from build123d import *

# Parameters (mm, degrees)
BOSS_EXTRUDE1_DEPTH  = 3.175
SKETCH2_W            = 107.95
SKETCH2_H            = 3.175
CUT_EXTRUDE1_DEPTH   = 355.989990176
SKETCH3_W            = 133.35
SKETCH3_H            = 19.05
CUT_EXTRUDE2_DEPTH   = 355.989990176
FILLET1_R            = 1.5875
CUT_EXTRUDE3_DEPTH   = 355.989990176
LPATTERN1_COUNT      = 2
LPATTERN1_PITCH      = 101.6
LPATTERN1_COUNT_DIR2 = 2
LPATTERN1_PITCH_DIR2 = 146.05
CUT_EXTRUDE4_DEPTH   = 355.989990176
FILLET2_R            = 1.5875


with BuildPart() as part:
    # Sketch1 → Boss-Extrude1 (new body)
    with BuildSketch(Plane(origin=(0, 0, 0), x_dir=(1, 0, 0), z_dir=(0, 1, 0))):
        Polygon((130.175, 0), (158.75, 0), (158.75, 317.5), (0, 317.5), (0, 0), (28.575, 0), (28.575, -3.175), (130.175, -3.175), align=None)
    extrude(amount=BOSS_EXTRUDE1_DEPTH)

    # Sketch2 → Cut-Extrude1 (cut, through all)
    with BuildSketch(Plane(origin=(0, 3.175, 0), x_dir=(1, 0, 0), z_dir=(0, 1, 0))):
        with Locations((79.375, 315.9125)):
            Rectangle(SKETCH2_W, SKETCH2_H)
    extrude(amount=-CUT_EXTRUDE1_DEPTH, mode=Mode.SUBTRACT)

    # Sketch3 → Cut-Extrude2 (cut, through all)
    with BuildSketch(Plane(origin=(0, 3.175, 0), x_dir=(1, 0, 0), z_dir=(0, 1, 0))):
        with Locations((79.375, 57.15)):
            Rectangle(SKETCH3_W, SKETCH3_H)
    extrude(amount=-CUT_EXTRUDE2_DEPTH, mode=Mode.SUBTRACT)

    # Fillet1
    fillet1_edges = [part.edges().sort_by_distance(p)[0] for p in [
        (25.4, 1.5875, -314.325),
        (25.4, 1.5875, -317.5),
        (0, 1.5875, -317.5),
        (0, 1.5875, 0),
        (28.575, 1.5875, 0),
        (28.575, 1.5875, 3.175),
        (130.175, 1.5875, 3.175),
        (130.175, 1.5875, 0),
        (158.75, 1.5875, 0),
        (158.75, 1.5875, -317.5),
        (133.35, 1.5875, -317.5),
        (133.35, 1.5875, -314.325),
    ]]
    fillet(fillet1_edges, radius=FILLET1_R - 0.0001)  # a hair under: the kernel refuses the full size

    # Sketch4 → Cut-Extrude3 (cut, through all)
    with BuildSketch(Plane(origin=(0, 3.175, 0), x_dir=(1, 0, 0), z_dir=(0, 1, 0))):
        with BuildLine():
            Line((4.445, 238.114159312), (4.445, 241.3))
            ThreePointArc((4.445, 241.3), (6.35, 243.205), (8.255, 241.3))
            Line((8.255, 241.3), (8.255, 238.114159312))
            ThreePointArc((8.255, 238.114159312), (6.35, 230.66375), (4.445, 238.114159312))
        make_face()
    cut_extrude3 = extrude(amount=-CUT_EXTRUDE3_DEPTH, mode=Mode.SUBTRACT)

    # LPattern1: Cut-Extrude3 2 × 2
    with Locations(*[(j * LPATTERN1_PITCH_DIR2, 0, i * LPATTERN1_PITCH) for i in range(LPATTERN1_COUNT) for j in range(LPATTERN1_COUNT_DIR2) if (i, j) != (0, 0)]):
        add(cut_extrude3, mode=Mode.SUBTRACT)

    # Sketch5 → Cut-Extrude4 (cut, through all)
    with BuildSketch(Plane(origin=(0, 3.175, 0), x_dir=(1, 0, 0), z_dir=(0, 1, 0))):
        Polygon((139.7, 111.125), (114.3, 85.725), (133.35, 85.725), (139.7, 92.075), align=None)
        Polygon((139.7, 149.225), (76.2, 85.725), (95.25, 85.725), (139.7, 130.175), align=None)
        Polygon((139.7, 187.325), (38.1, 85.725), (57.15, 85.725), (139.7, 168.275), align=None)
        Polygon((19.05, 104.775), (19.05, 85.725), (139.7, 206.375), (139.7, 225.425), align=None)
        Polygon((19.05, 142.875), (19.05, 123.825), (139.7, 244.475), (139.7, 263.525), align=None)
        Polygon((19.05, 180.975), (19.05, 161.925), (139.7, 282.575), (139.7, 295.275), (133.35, 295.275), align=None)
        Polygon((19.05, 219.075), (19.05, 200.025), (114.3, 295.275), (95.25, 295.275), align=None)
        Polygon((19.05, 257.175), (19.05, 238.125), (76.2, 295.275), (57.15, 295.275), align=None)
        Polygon((19.05, 295.275), (19.05, 276.225), (38.1, 295.275), align=None)
    extrude(amount=-CUT_EXTRUDE4_DEPTH, mode=Mode.SUBTRACT)

    # Fillet2
    fillet2_edges = [part.edges().sort_by_distance(p)[0] for p in [
        (19.05, 1.5875, -104.775),
        (139.7, 1.5875, -225.425),
        (139.7, 1.5875, -206.375),
        (19.05, 1.5875, -85.725),
        (19.05, 1.5875, -142.875),
        (139.7, 1.5875, -263.525),
        (139.7, 1.5875, -244.475),
        (19.05, 1.5875, -123.825),
        (95.25, 1.5875, -85.725),
        (76.2, 1.5875, -85.725),
        (139.7, 1.5875, -149.225),
        (139.7, 1.5875, -130.175),
        (57.15, 1.5875, -85.725),
        (38.1, 1.5875, -85.725),
        (139.7, 1.5875, -187.325),
        (139.7, 1.5875, -168.275),
        (19.05, 1.5875, -257.175),
        (57.15, 1.5875, -295.275),
        (76.2, 1.5875, -295.275),
        (19.05, 1.5875, -238.125),
        (19.05, 1.5875, -276.225),
        (19.05, 1.5875, -295.275),
        (38.1, 1.5875, -295.275),
        (19.05, 1.5875, -180.975),
        (133.35, 1.5875, -295.275),
        (139.7, 1.5875, -295.275),
        (139.7, 1.5875, -282.575),
        (19.05, 1.5875, -161.925),
        (19.05, 1.5875, -219.075),
        (95.25, 1.5875, -295.275),
        (114.3, 1.5875, -295.275),
        (19.05, 1.5875, -200.025),
        (133.35, 1.5875, -85.725),
        (114.3, 1.5875, -85.725),
        (139.7, 1.5875, -111.125),
        (139.7, 1.5875, -92.075),
    ]]
    fillet(fillet2_edges, radius=FILLET2_R)


solid = part.part
Can you work these out from the model? Positions are in its coordinate system, mm. Give positions to 0.01 mm unless a question says otherwise; leave off trailing zeros. Loops run counter-clockwise (first coordinate to the right, second up) from the corner with the lowest first, then second, coordinate; pieces in that order, holes last. Notation, with made-up numbers: (69, -3.5) -> (93, -3.5) arc R17 ccw to (93, 11.5) -> close; hole circle Ø11 at (32, 75.25). An arc over 180 degrees is marked (long way). Write item = value, one per line.
1) Will this pin go through, and if not, where does the flat tip stop? pin 1 (3 mm diameter, centred on x = 134, z = -32, fed in from -Y).
Check result:
pin_1 = 0
2) Suppose I cut it at B-B on z = -150. Write out the boundary of the cut face in (x, y) (3 decimals).
Check result:
outline = (0, 0) -> (26.175, 0) -> (26.175, 3.175) -> (0, 3.175) -> close; (45.225, 0) -> (64.275, 0) -> (64.275, 3.175) -> (45.225, 3.175) -> close; (83.325, 0) -> (102.375, 0) -> (102.375, 3.175) -> (83.325, 3.175) -> close; (121.425, 0) -> (158.75, 0) -> (158.75, 3.175) -> (121.425, 3.175) -> close
3) Thinking about a two-plate mould opening in X: for faces 1 (the flat face through (79.675, 1.61, -222.55)), 2 (the flat face through (61, 3.175, -159)), which applies, released by +X, released by -X, zero draft, split by the parting line, or undercut?
Check result:
face_1 = undercut
face_2 = zero draft
4) Suppose I cut it at A-A on x = 51.5. Give the number of separate pieces and of enclosed holes in the cut face, then the cut area to 3 significant figures.
Check result:
separate_pieces = 8
enclosed_holes = 0
area = 603 mm2
5) I need wall thicknesses on L1, parallel to Z at x = 152.4, y = 2.2 (3 decimals); L2, parallel to X at y = 0.65, z = -292.5 (3 decimals); L3, parallel to X at y = 2.7, z = -126 (3 decimals). Which ranges of each line are inside material? Lowest first, please. Write a range as from..to.
Check result:
L1 = -317.5..-243.205, -230.664..-141.605, -129.064..0
L2 = 0..19.05, 35.325..54.375, 73.425..92.475, 111.525..130.575, 139.7..158.75
L3 = 0..40.275, 59.325..78.375, 97.425..116.475, 135.525..158.75
